Autodesk Inventor part; units mm, degrees
ref_plane "YZ Plane" through (0, 0, 0) normal (1, 0, 0) x (0, 1, 0)
ref_plane "XZ Plane" through (0, 0, 0) normal (0, 1, 0) x (-1, 0, 0)
ref_plane "XY Plane" through (0, 0, 0) normal (0, 0, 1) x (1, 0, 0)
sketch "スケッチ1" plane through (0, 0, 0) normal (0, 0, 1) x (1, 0, 0)
  circle A0 centre (0, 5) radius 1.55
  circle A1 centre (0, -5) radius 1.55
  line L0 (0, 5) -> (0, -5) construction
  line L1 (0, 0) -> (100, 0) construction
  circle A2 centre (100, 0) radius 1.55
  line L2 (-5, 10) -> (-5, -10)
  line L3 (-5, -10) -> (5, -10)
  line L4 (5, -10) -> (100.2521, -5.9947)
  line L5 (-5, 10) -> (5, 10)
  line L6 (5, 10) -> (100.2521, 5.9947)
  arc A3 (100.2521, -5.9947) -> (100.2521, 5.9947) centre (100, 0) ccw
  circle A4 centre (0, 5) radius 3 construction
  circle A5 centre (0, 5) radius 5 construction
  line L7 (5, 10) -> (5, -10) construction
  point P0 (-5, 0)
  dimension "d0" = 10
  dimension "d1" = 3.1
  dimension "d2" = 3.1
  dimension "d3" = 100
  dimension "d4" = 6
  dimension "d5" = 6
  dimension "d6" = 2
extrude "押し出し1" add sketch "スケッチ1" along normal blind 5
sketch "スケッチ2" plane through (0, 0, 0) normal (0, 0, -1) x (-1, 0, 0)
  circle A0 centre (-100, 0) radius 1.55
  arc A1 (-100.2521, 5.9947) -> (-100.2521, -5.9947) centre (-100, 0) ccw
  circle A2 centre (-100, 0) radius 4.05
  point P0 (0, 0)
  dimension "d9" = 8.1
extrude "押し出し2" cut sketch "スケッチ2" against normal blind 3
sketch "スケッチ3" plane through (0, 0, 0) normal (0, 0, -1) x (-1, 0, 0)
  circle A0 centre (0, -5) radius 1.55
  circle A1 centre (0, 5) radius 1.55
  line L0 (0, -1.8246) -> (2.75, -3.4123)
  line L1 (2.75, -3.4123) -> (2.75, -6.5877)
  line L2 (2.75, -6.5877) -> (0, -8.1754)
  line L3 (0, -8.1754) -> (-2.75, -6.5877)
  line L4 (-2.75, -6.5877) -> (-2.75, -3.4123)
  line L5 (-2.75, -3.4123) -> (0, -1.8246)
  line L6 (-2.75, 6.5877) -> (0, 8.1754)
  line L7 (0, 8.1754) -> (2.75, 6.5877)
  line L8 (2.75, 6.5877) -> (2.75, 3.4123)
  line L9 (2.75, 3.4123) -> (0, 1.8246)
  line L10 (0, 1.8246) -> (-2.75, 3.4123)
  line L11 (-2.75, 3.4123) -> (-2.75, 6.5877)
  line L12 (0, -8.2332) -> (2.8, -6.6166)
  line L13 (2.8, -6.6166) -> (2.8, -3.3834)
  line L14 (2.8, -3.3834) -> (0, -1.7668)
  line L15 (0, -1.7668) -> (-2.8, -3.3834)
  line L16 (-2.8, -3.3834) -> (-2.8, -6.6166)
  line L17 (-2.8, -6.6166) -> (0, -8.2332)
  line L18 (-2.8, 3.3834) -> (0, 1.7668)
  line L19 (0, 1.7668) -> (2.8, 3.3834)
  line L20 (2.8, 3.3834) -> (2.8, 6.6166)
  line L21 (2.8, 6.6166) -> (0, 8.2332)
  line L22 (0, 8.2332) -> (-2.8, 6.6166)
  line L23 (-2.8, 6.6166) -> (-2.8, 3.3834)
  circle A2 centre (0, -7.1832) radius 1.05
  circle A3 centre (1.8907, -6.0916) radius 1.05
  circle A4 centre (1.8907, -3.9084) radius 1.05
  circle A5 centre (0, -2.8168) radius 1.05
  circle A6 centre (-1.8907, -3.9084) radius 1.05
  circle A7 centre (-1.8907, -6.0916) radius 1.05
  circle A8 centre (0, 2.8168) radius 1.05
  circle A9 centre (1.8907, 3.9084) radius 1.05
  circle A10 centre (1.8907, 6.0916) radius 1.05
  circle A11 centre (0, 7.1832) radius 1.05
  circle A12 centre (-1.8907, 6.0916) radius 1.05
  circle A13 centre (-1.8907, 3.9084) radius 1.05
  point P0 (0, 0)
  point P1 (2.8, -6.6166)
  point P2 (2.8, -3.3834)
  point P3 (0, -1.7668)
  point P4 (-2.8, -3.3834)
  point P5 (-2.8, -6.6166)
  point P6 (2.8, 3.3834)
  point P7 (2.8, 6.6166)
  point P8 (0, 8.2332)
  point P9 (-2.8, 6.6166)
  point P10 (-2.8, 3.3834)
  dimension "d16" = 2.1
  dimension "d15" = 5.5
  dimension "d17" = 0.05
  dimension "d20" = 360
  dimension "d24" = 360
extrude "押し出し3" cut sketch "スケッチ3" against normal blind 1
sketch "スケッチ4" plane through (0, 0, 0) normal (0, 0, -1) x (-1, 0, 0)
  circle A0 centre (-100, 0) radius 4.05
  line L0 (-100.2521, 5.9947) -> (-5, 10)
  arc A1 (-100.2521, 5.9947) -> (-100.2521, -5.9947) centre (-100, 0) ccw
  line L1 (-5, -10) -> (-100.2521, -5.9947)
  line L2 (-7.8, -6.8796) -> (-94.9345, -3.2157)
  line L3 (-5, -10) -> (-100.2521, -5.9947)
  arc A2 (-94.9345, -3.2157) -> (-94.9345, 3.2157) centre (-100, 0) ccw
  line L4 (-94.9345, 3.2157) -> (-7.8, 6.8796)
  line L5 (-7.8, 6.8796) -> (-7.8, -6.8796)
  point P0 (-2.8, 4.4334)
  point P1 (0, 0)
  dimension "d26" = 3
  dimension "d27" = 3
  dimension "d28" = 5
extrude "押し出し4" cut sketch "スケッチ4" against normal blind 4 contours L2 A2 L4 L5
fillet "フィレット1" radius 2 4 edges at (7.8, 6.8796, 2) (7.8, -6.8796, 2) (94.9345, 3.2157, 2) (94.9345, -3.2157, 2)
equation "\"d27\" = d26"
properties part number "胴体_サブフレーム_1_12" material "アセタール樹脂、黒"
Geometry check sheet. Reference: the model listing, model coordinates, mm. A direction names the side the tool comes from. Give positions to 0.01 mm unless a question says otherwise; leave off trailing zeros. Loops run counter-clockwise (first coordinate to the right, second up) from the corner with the lowest first, then second, coordinate; pieces in that order, holes last. Notation, with made-up numbers: (31, 32.25) -> (67, 32.25) arc R11 ccw to (67, 45.25) -> close; hole circle Ø5 at (49.5, -8.5). An arc over 180 degrees is marked (long way). Answer in a Markdown table with one row per item. Add a question column.
1) Material ranges on probe 1 along Y at (x, z) = (0, 4.05); probe 2 along Y at (x, z) = (100, 3.75); probe 3 along Y at (x, z) = (100, 1.85), recorded low to high. Write a range as from..to.
2) Cross-section at B-B on y = 0. Record the boundary of the cut face in (x, z).
3) Cross-section at C-C on z = 1.9. Record the boundary of the cut face in (x, y).
4) Draft check along Y on faces 1 (the face through (51.616, 5.037, 1.972)), 2 (the face through (0, -10, 2)), 3 (the face through (-5, 0, 2)). Enter one of: pulls with the +Y half, pulls with the -Y half, needs draft (parallel to the pull), parting line crosses it, or undercut.
5) Cross-section at D-D on x = 72.5. Record the boundary of the cut face in (y, z).
6) Gauge pin test, flat ends, axial feed: P1, Ø1, axis at x = 36, z = 3, coming from the -Y side; P2, Ø4, axis at x = 0, y = -5, coming from the +Z side; P3, Ø2.5, axis at x = 98.5, y = 0.5, coming from the -Z side; P4, Ø1.1, axis at y = 5, z = 0.5, coming from the +X side. Record the tip position at first contact, or that the pin passes through.
7) Cross-section at A-A on x = 0. Record the boundary of the cut face in (y, z).
8) Set-up check for faces 4 (the face through (106, 0, 2)), 5 (the face through (7.8, 0, 2)): record each of +Z, -Z, +X, -X, +Y, -Y from which the full face is reachable in a straight line by a thin tool's end or side.
Outcome:
| question | item | result |
|---|---|---|
| 1 | probe 1 | y = -10..-6.55, -3.45..3.45, 6.55..10 |
| 1 | probe 2 | y = -6.01..-1.55, 1.55..6.01 |
| 1 | probe 3 | y = -6.01..-4.05, 4.05..6.01 |
| 2 | outline | (-5, 0) -> (7.8, 0) -> (7.8, 4) -> (94, 4) -> (94, 0) -> (95.95, 0) -> (95.95, 3) -> (98.45, 3) -> (98.45, 5) -> (-5, 5) -> close; (101.55, 3) -> (104.05, 3) -> (104.05, 0) -> (106, 0) -> (106, 5) -> (101.55, 5) -> close |
| 3 | outline | (-5, -10) -> (5, -10) -> (100.25, -5.99) arc R6 ccw to (100.25, 5.99) -> (5, 10) -> (-5, 10) -> close; hole circle Ø3.1 at (0, -5); hole circle Ø3.1 at (0, 5); hole (7.8, -4.79) arc R2 ccw to (9.88, -6.79) -> (92.2, -3.33) arc R2 ccw to (94.08, -1) arc R6 cw to (94.08, 1) arc R2 ccw to (92.2, 3.33) -> (9.88, 6.79) arc R2 ccw to (7.8, 4.79) -> close; hole circle Ø8.1 at (100, 0) |
| 4 | face 1 | undercut |
| 4 | face 2 | pulls with the -Y half |
| 4 | face 3 | needs draft |
| 5 | outline | (-7.16, 0) -> (-4.16, 0) -> (-4.16, 4) -> (4.16, 4) -> (4.16, 0) -> (7.16, 0) -> (7.16, 5) -> (-7.16, 5) -> close |
| 6 | P1 | stops at y = -8.72 |
| 6 | P2 | stops at z = 5 |
| 6 | P3 | stops at z = 3 |
| 6 | P4 | stops at x = 104.02 |
| 7 | outline | (-10, 0) -> (-8.23, 0) -> (-8.23, 1) -> (-6.55, 1) -> (-6.55, 5) -> (-10, 5) -> close; (-3.45, 1) -> (-1.77, 1) -> (-1.77, 0) -> (1.77, 0) -> (1.77, 1) -> (3.45, 1) -> (3.45, 5) -> (-3.45, 5) -> close; (6.55, 1) -> (8.23, 1) -> (8.23, 0) -> (10, 0) -> (10, 5) -> (6.55, 5) -> close |
| 8 | face 4 | +Z, -Z, +X |
| 8 | face 5 | -Z |
